from build123d import *

# Parameters (mm, degrees)
SKETCH1_R           = 32.5
BOSS_EXTRUDE1_DEPTH = 6
SKETCH16_R          = 1.1
CUT_EXTRUDE8_DEPTH  = 47.351914739
SKETCH17_R          = 2
CUT_EXTRUDE9_DEPTH  = 2.4
SKETCH12_R          = 1.65
CUT_EXTRUDE10_DEPTH = 47.351914739


with BuildPart() as part:
    # Sketch1 → Boss-Extrude1 (new body)
    with BuildSketch(Plane.XY):
        Circle(SKETCH1_R)
    extrude(amount=BOSS_EXTRUDE1_DEPTH)

    # Sketch16 → Cut-Extrude8 (cut, through all)
    with BuildSketch(Plane.XY.offset(6)):
        with Locations((8, 0)):
            Circle(SKETCH16_R)
        with Locations((-8, 0)):
            Circle(SKETCH16_R)
        with Locations((0, -8)):
            Circle(SKETCH16_R)
        with Locations((0, 8)):
            Circle(SKETCH16_R)
    extrude(amount=-CUT_EXTRUDE8_DEPTH, mode=Mode.SUBTRACT)

    # Sketch17 → Cut-Extrude9 (cut)
    with BuildSketch(Plane.XY.offset(6)):
        with Locations((8, 0)):
            Circle(SKETCH17_R)
        with Locations((-8, 0)):
            Circle(SKETCH17_R)
        with Locations((0, -8)):
            Circle(SKETCH17_R)
        with Locations((0, 8)):
            Circle(SKETCH17_R)
    extrude(amount=-CUT_EXTRUDE9_DEPTH, mode=Mode.SUBTRACT)

    # Sketch12 → Cut-Extrude10 (cut, through all)
    with BuildSketch(Plane.XY.offset(6)):
        with Locations((0, 25)):
            Circle(SKETCH12_R)
        with Locations((25, 0)):
            Circle(SKETCH12_R)
        with Locations((0, -25)):
            Circle(SKETCH12_R)
        with Locations((-25, 0)):
            Circle(SKETCH12_R)
    extrude(amount=-CUT_EXTRUDE10_DEPTH, mode=Mode.SUBTRACT)


solid = part.part
Geometry check sheet. Reference: the model listing, model coordinates, mm. A direction names the side the tool comes from. Give positions to 0.01 mm unless a question says otherwise; leave off trailing zeros. Order: outer loops, then holes, each group sorted by start corner. A loop starts at its lowest first (then second) coordinate and runs counter-clockwise, first axis right, second up. Notation, with made-up numbers: (88, 69.25) - (136, 69.25) arc R29 ccw to (136, 106.25) - close; hole circle Ø5 at (70, 82.25). An arc over 180 degrees is marked (long way). Answer as a JSON object with one key per item and string values.
(1) Cross-section at A-A (z = 0.8). State how many separate pieces and enclosed holes the cut face has, then the cut area to 3 significant figures.
Report:
{"separate pieces": "1", "enclosed holes": "8", "area": "3,270 mm^2"}
(2) Depth check by flat-ended pin: pin 1 Ø2.5 at (x, y) = (25, 0) entering from +Z; pin 2 Ø1.5 at (y, z) = (-18.5, 1) entering from +X; pin 3 Ø1.2 at (x, y) = (-1, 8.5) entering from +Z; pin 4 Ø5.5 at (x, y) = (0, 25) entering from -Z. Enter the tip coordinate at first touch or a pass-through.
Report:
{"pin 1": "through", "pin 2": "x = 27.22", "pin 3": "z = 3.6", "pin 4": "z = 0"}
(3) Draft check along X on faces 3 (the cylindrical face through (0, -6, 5)), 4 (the cylindrical face through (31, 9.76, 2.96)), 5 (the flat face through (0, 0, 0)), 6 (the cylindrical face through (-0.238, 6.926, 1.825)). Enter one of: released by +X, released by -X, zero draft, split by the parting line, or undercut.
Report:
{"face 3": "undercut", "face 4": "split by the parting line", "face 5": "zero draft", "face 6": "undercut"}
(4) Cross-section at D-D (x = -25). Record the cut outline in (y, z).
Report:
{"outline": "(-20.77, 0) - (-1.65, 0) - (-1.65, 6) - (-20.77, 6) - close; (1.65, 0) - (20.77, 0) - (20.77, 6) - (1.65, 6) - close"}
(5) Material ranges on line 1 (Y direction, x = 0, z = 5.15); line 2 (Y direction, x = -0.5, z = 4.2); line 3 (Y direction, x = 8, z = 1.1), recorded low to high.
Report:
{"line 1": "-32.5 to -26.65, -23.35 to -10, -6 to 6, 10 to 23.35, 26.65 to 32.5", "line 2": "-32.5 to -26.57, -23.43 to -9.94, -6.06 to 6.06, 9.94 to 23.43, 26.57 to 32.5", "line 3": "-31.5 to -1.1, 1.1 to 31.5"}
(6) Cross-section at C-C (x = 0). Record the cut outline in (y, z), then the cut area to 3 significant figures.
Report:
{"outline": "(-32.5, 0) - (-26.65, 0) - (-26.65, 6) - (-32.5, 6) - close; (-23.35, 0) - (-9.1, 0) - (-9.1, 3.6) - (-10, 3.6) - (-10, 6) - (-23.35, 6) - close; (-6.9, 0) - (6.9, 0) - (6.9, 3.6) - (6, 3.6) - (6, 6) - (-6, 6) - (-6, 3.6) - (-6.9, 3.6) - close; (9.1, 0) - (23.35, 0) - (23.35, 6) - (10, 6) - (10, 3.6) - (9.1, 3.6) - close; (26.65, 0) - (32.5, 0) - (32.5, 6) - (26.65, 6) - close", "area": "315 mm^2"}
(7) Tool access check on faces 1 (the cylindrical face through (6, 0, 5)), 2 (the cylindrical face through (-6.984, -0.421, 1.825)). Record the directions out of +Z, -Z, +X, -X, +Y, -Y that give a thin tool (end or side, any length) a straight path to the whole face; none if there is none.
Report:
{"face 1": "+Z", "face 2": "+Z, -Z"}
(8) Cross-section at B-B (y = 8). Record the cut outline in (x, z), then the cut area to 3 significant figures.
Report:
{"outline": "(-31.5, 0) - (-1.1, 0) - (-1.1, 3.6) - (-2, 3.6) - (-2, 6) - (-31.5, 6) - close; (1.1, 0) - (31.5, 0) - (31.5, 6) - (2, 6) - (2, 3.6) - (1.1, 3.6) - close", "area": "360 mm^2"}
